Geometry check sheet. Reference: the model listing, model coordinates, mm. Round coordinates to 2 decimals unless told otherwise and drop trailing zeros. Loops run counter-clockwise (first coordinate to the right, second up) from the corner with the lowest first, then second, coordinate; pieces in that order, holes last. Notation, with made-up numbers: (71.5, -32.5) - (80.5, -32.5) arc R19 cw to (80.5, -8.5) - close; hole circle Ø11 at (28.25, 10.5). An arc over 180 degrees is marked (long way). Write item = value, one per line.
```python
from build123d import *

# Parameters (mm, degrees)
SKETCH1_R           = 1.4
BOSS_EXTRUDE1_DEPTH = 2


with BuildPart() as part:
    # Sketch1 → Boss-Extrude1 (new body)
    with BuildSketch(Plane.XY):
        with BuildLine():
            Line((-1.5, -3.4), (-1.5, -1.4))
            Line((-1.5, -1.4), (-1.5, 3.6))
            Line((-1.5, 3.6), (-1.5, 11.6))
            Line((-1.5, 11.6), (3.099578521, 1.397359292))
            ThreePointArc((3.099578521, 1.397359292), (2.855785495, -1.845125796), (0, -3.4))
            Line((0, -3.4), (-1.5, -3.4))
        make_face()
        Circle(SKETCH1_R, mode=Mode.SUBTRACT)
    extrude(amount=BOSS_EXTRUDE1_DEPTH)


solid = part.part
```
(1) Gauge pin test, flat end, axial feed: pin 1 (1 mm diameter, centred on x = -0.5, y = 0, fed in from +Z). Record the tip position at first contact, or that the pin passes through.
Answers follow:
pin_1 = through
(2) Mould release check, pull along X, two halves, no side actions. Record for faces 1 (the cylindrical face through (1.335, 0.421, 0.986)), 2 (the flat face through (0.768, 6.57, 0.986)), 3 (the flat face through (0, 3, 0)), 4 (the flat face through (-1.5, 4, 1)): pulls with the +X half, pulls with the -X half, needs draft (parallel to the pull), parting line crosses it, or undercut.
Answers follow:
face_1 = undercut
face_2 = pulls with the +X half
face_3 = needs draft
face_4 = pulls with the -X half
(3) Scan lines: L1, parallel to Y at x = -0.3, z = 0.65; L2, parallel to Y at x = 0, z = 1; L3, parallel to X at y = -1.25, z = 1.4. Record each from-to range of solid material in increasing order. Write a range as [from, to].
Answers follow:
L1 = [-3.4, -1.37], [1.37, 8.94]
L2 = [-3.4, -1.4], [1.4, 8.27]
L3 = [-1.5, -0.63], [0.63, 3.16]
(4) Section check B-B (x = -1). Enter the section's corners in (y, z).
Answers follow:
outline = (-3.4, 0) - (-0.98, 0) - (-0.98, 2) - (-3.4, 2) - close; (0.98, 0) - (10.49, 0) - (10.49, 2) - (0.98, 2) - close
(5) Section check C-C (z = 0.15). Enter the section's corners in (x, y), then the cut area to 3 significant figures.
Answers follow:
outline = (-1.5, -3.4) - (0, -3.4) arc R3.4 ccw to (3.1, 1.4) - (-1.5, 11.6) - close; hole circle Ø2.8 at (0, 0)
area = 38.2 mm²
(6) Section check A-A (y = 0). Enter the section's corners in (x, z), then the cut area to 3 significant figures.
Answers follow:
outline = (-1.5, 0) - (-1.4, 0) - (-1.4, 2) - (-1.5, 2) - close; (1.4, 0) - (3.4, 0) - (3.4, 2) - (1.4, 2) - close
area = 4.20 mm²
(7) Section check D-D (x = 2.65). Enter the section's corners in (y, z).
Answers follow:
outline = (-2.13, 0) - (2.39, 0) - (2.39, 2) - (-2.13, 2) - close
